from build123d import *

# Parameters (mm, degrees)
SKETCH1_W           = 60.33
SKETCH1_H           = 4
BOSS_EXTRUDE1_DEPTH = 30
FILLET1_SIZE        = 15
FILLET2_SIZE        = 3


with BuildPart() as part:
    # Sketch1 → Boss-Extrude1 (new body)
    with BuildSketch(Plane.XY):
        Polygon((-36.165, 0), (-30.165, 0), (-30.165, 4), (-30.165, 25), (-36.165, 25), align=None)
        Polygon((-30.165, -4), (-30.165, 0), (-36.165, 0), (-36.165, -25), (-30.165, -25), align=None)
        with Locations((0, -2)):
            Rectangle(SKETCH1_W, SKETCH1_H)
        with Locations((0, 2)):
            Rectangle(SKETCH1_W, SKETCH1_H)
        Polygon((30.165, 0), (36.165, 0), (36.165, 25), (30.165, 25), (30.165, 4), align=None)
        Polygon((36.165, -25), (36.165, 0), (30.165, 0), (30.165, -4), (30.165, -25), align=None)
    extrude(amount=BOSS_EXTRUDE1_DEPTH)

    # Fillet1
    # a fillet whose section is not a circle: 15 mm, written as the material it adds along each edge
    with BuildSketch(Plane(origin=(30.165, -4, 0), x_dir=(0, -1, 0), z_dir=(0, 0, 1)), Plane(origin=(30.165, 4, 0), x_dir=(-1, 0, 0), z_dir=(0, 0, 1)), Plane(origin=(-30.165, -4, 0), x_dir=(1, 0, 0), z_dir=(0, 0, 1))) as fillet1_piece_1:
        with BuildLine():
            add(Edge.make_bspline([(FILLET1_SIZE, 0), (FILLET1_SIZE * 0.831801948466, 0), (FILLET1_SIZE * 0.663603896932, 0), (FILLET1_SIZE * 0.292893218813, -FILLET1_SIZE * 0.0716919198361), (FILLET1_SIZE * 0.0716919198361, -FILLET1_SIZE * 0.292893218813), (0, -FILLET1_SIZE * 0.663603896932), (0, -FILLET1_SIZE * 0.831801948466), (0, -FILLET1_SIZE)], knots=[0, 0, 0, 0, 0, 0, 0.5, 0.5, 1, 1, 1, 1, 1, 1], degree=5))
            Line((0, -FILLET1_SIZE), (-FILLET1_SIZE * 0.02, -FILLET1_SIZE))
            Line((-FILLET1_SIZE * 0.02, -FILLET1_SIZE), (-FILLET1_SIZE * 0.02, FILLET1_SIZE * 0.02))
            Line((-FILLET1_SIZE * 0.02, FILLET1_SIZE * 0.02), (FILLET1_SIZE, FILLET1_SIZE * 0.02))
            Line((FILLET1_SIZE, FILLET1_SIZE * 0.02), (FILLET1_SIZE, 0))
        make_face()
    extrude(amount=30)
    with BuildSketch(Plane(origin=(-30.165, 4, 0), x_dir=(1, 0, 0), z_dir=(0, 0, 1))) as fillet1_piece_2:
        with BuildLine():
            add(Edge.make_bspline([(FILLET1_SIZE, 0), (FILLET1_SIZE * 0.831801948466, 0), (FILLET1_SIZE * 0.663603896932, 0), (FILLET1_SIZE * 0.292893218813, FILLET1_SIZE * 0.0716919198361), (FILLET1_SIZE * 0.0716919198361, FILLET1_SIZE * 0.292893218813), (0, FILLET1_SIZE * 0.663603896932), (0, FILLET1_SIZE * 0.831801948466), (0, FILLET1_SIZE)], knots=[0, 0, 0, 0, 0, 0, 0.5, 0.5, 1, 1, 1, 1, 1, 1], degree=5))
            Line((0, FILLET1_SIZE), (-FILLET1_SIZE * 0.02, FILLET1_SIZE))
            Line((-FILLET1_SIZE * 0.02, FILLET1_SIZE), (-FILLET1_SIZE * 0.02, -FILLET1_SIZE * 0.02))
            Line((-FILLET1_SIZE * 0.02, -FILLET1_SIZE * 0.02), (FILLET1_SIZE, -FILLET1_SIZE * 0.02))
            Line((FILLET1_SIZE, -FILLET1_SIZE * 0.02), (FILLET1_SIZE, 0))
        make_face()
    extrude(amount=30)

    # Fillet2
    # a fillet whose section is not a circle: 3 mm, written as the material it takes off along each edge
    with BuildSketch(Plane(origin=(30.165, 25, -7.5), x_dir=(1, 0, 0), z_dir=(0, 0, 1)), Plane(origin=(36.165, 25, -7.5), x_dir=(0, -1, 0), z_dir=(0, 0, 1)), Plane(origin=(36.165, -25, -7.5), x_dir=(-1, 0, 0), z_dir=(0, 0, 1)), Plane(origin=(30.165, -25, -7.5), x_dir=(0, 1, 0), z_dir=(0, 0, 1)), Plane(origin=(-30.165, -25, -7.5), x_dir=(-1, 0, 0), z_dir=(0, 0, 1)), Plane(origin=(-36.165, -25, -7.5), x_dir=(0, 1, 0), z_dir=(0, 0, 1)), Plane(origin=(-36.165, 25, -7.5), x_dir=(1, 0, 0), z_dir=(0, 0, 1)), Plane(origin=(-30.165, 25, -7.5), x_dir=(0, -1, 0), z_dir=(0, 0, 1))) as fillet2_piece_1:
        with BuildLine():
            add(Edge.make_bspline([(FILLET2_SIZE, 0), (FILLET2_SIZE * 0.831801948466, 0), (FILLET2_SIZE * 0.663603896932, 0), (FILLET2_SIZE * 0.292893218813, -FILLET2_SIZE * 0.0716919198361), (FILLET2_SIZE * 0.0716919198361, -FILLET2_SIZE * 0.292893218813), (0, -FILLET2_SIZE * 0.663603896932), (0, -FILLET2_SIZE * 0.831801948466), (0, -FILLET2_SIZE)], knots=[0, 0, 0, 0, 0, 0, 0.5, 0.5, 1, 1, 1, 1, 1, 1], degree=5))
            Line((0, -FILLET2_SIZE), (0, 0))
            Line((0, 0), (FILLET2_SIZE, 0))
        make_face()
    extrude(amount=45, mode=Mode.SUBTRACT)


solid = part.part
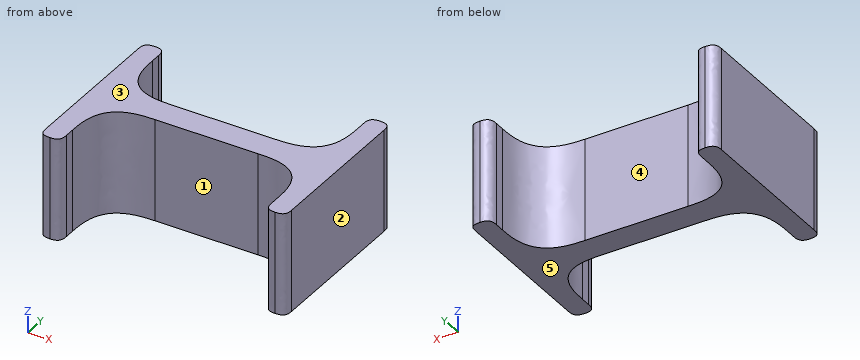
Input: part model. Units: mm. Frame: model coordinates. Face numbers are marked on the shaded views. A direction names the side the tool comes from. Give positions to 0.01 mm unless a question says otherwise; leave off trailing zeros. Loops run counter-clockwise (first coordinate to the right, second up) from the corner with the lowest first, then second, coordinate; pieces in that order, holes last. Notation, with made-up numbers: M -1,84.5 L 50,84.5 A19 ccw 50,105.5 Z; hole C 29,53 d11. An arc over 180 degrees is marked long. Use one line per item in the form item = value.
1. First-contact query: pin 1 (2 mm diameter, centred on x = -21, z = 8, fed in from +Y); pin 2 (1 mm diameter, centred on x = 26.5, z = 12.5, fed in from -Y); pin 3 (3 mm diameter, centred on x = -21, z = 26, fed in from +Y). Flat tips, straight axial feed; report the tip coordinate or a pass-through.
Numbers:
pin_1 = 4.65
pin_2 = -7.43
pin_3 = 4.79
2. Section query A-A, the plane x = 7. Return the cut outline in (y, z).
Numbers:
outline = M -4,0 L 4,0 L 4,30 L -4,30 Z
3. Pull-direction query (X, two-part tool) for the marked faces 1, 2 and 3; classes: released by +X, released by -X, zero draft, split by the parting line, or undercut.
Numbers:
face_1 = undercut
face_2 = released by +X
face_3 = zero draft
4. Line query: L1, parallel to X at y = -17.5, z = 21 (3 decimals); L2, parallel to Y at x = 1.5, z = 18; L3, parallel to X at y = 11, z = 15 (3 decimals). Output: solid intervals per line, ascending.
Numbers:
L1 = -36.165 to -30.157, 30.157 to 36.165
L2 = -4 to 4
L3 = -36.165 to -29.153, 29.153 to 36.165
5. Reachability of the marked faces 4 and 5 from +Z, -Z, +X, -X, +Y, -Y: full face, straight path, thin tool, end or side. Return the list, or none.
Numbers:
face_4 = +Z, -Z, +Y
face_5 = -Z, +X, -X, +Y, -Y
